from build123d import *

# Parameters (mm, degrees)
F1_DEPTH = 40
F3_DEPTH = 35
F4_R     = 35
F4_R_2   = 2
F5_DEPTH = 5


with BuildPart() as f1:
    # F0 (on Front) → F1 (new body, symmetric)
    with BuildSketch(Plane.XZ):
        Polygon((66.8717782649, 24.1746824527), (40.8910161514, 9.1746824527), (-28.3910161514, -30.8253175473), (-28.3910161514, -40.8253175473), (51.6089838486, -40.8253175473), (51.6089838486, -13.5048094716), (82.2307621135, 4.1746824527), (147.2307621135, 4.1746824527), (147.2307621135, 24.1746824527), align=None)
    extrude(amount=F1_DEPTH, both=True)

    # F2 (on Front) → F3 (cut, symmetric)
    with BuildSketch(Plane.XZ):
        with BuildLine():
            ThreePointArc((-23.4223891848, -30.2660805074), (17.6554756717, -37.2808918374), (50.6089838486, -11.772758664))
            Line((50.6089838486, -11.772758664), (81.6948637287, 6.1746824527))
            Line((81.6948637287, 6.1746824527), (145.2307621135, 6.1746824527))
            Line((145.2307621135, 6.1746824527), (145.2307621135, 12.1746824527))
            ThreePointArc((145.2307621135, 12.1746824527), (142.3018299254, 19.2457502646), (135.2307621135, 22.1746824527))
            Line((135.2307621135, 22.1746824527), (67.4076766498, 22.1746824527))
            Line((67.4076766498, 22.1746824527), (-23.4223891848, -30.2660805074))
        make_face()
    extrude(amount=F3_DEPTH, both=True, mode=Mode.SUBTRACT)

    # F4 (on face) → F5 (cut)
    with BuildSketch(Plane(origin=(6.25, 0, -10.8253175473), x_dir=(0.8660254038, 0, 0.5), z_dir=(-0.5, 0, 0.8660254038))):
        Circle(F4_R)
        with Locations((-35.75, 35.75)):
            Circle(F4_R_2)
        with Locations((35.75, 35.75)):
            Circle(F4_R_2)
        with Locations((35.75, -35.75)):
            Circle(F4_R_2)
        with Locations((-35.75, -35.75)):
            Circle(F4_R_2)
    extrude(amount=-F5_DEPTH, mode=Mode.SUBTRACT)


solid = f1.part
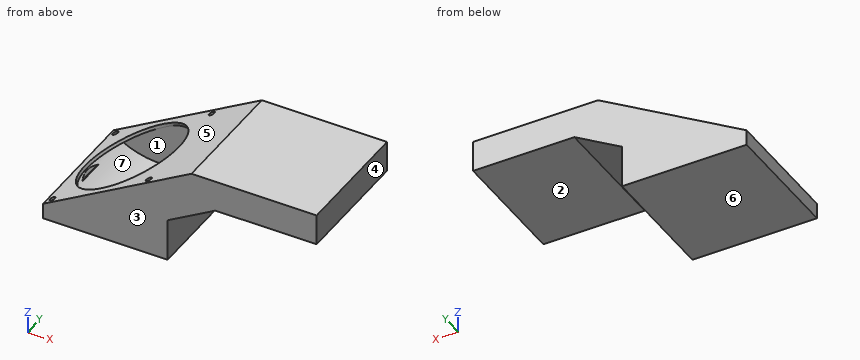
The listing builds one solid part. Answer for the finished solid, in the listing's coordinates (mm). Face numbers are marked on the shaded views. A direction names the side the tool comes from. Coordinates: 2 decimals unless noted, no trailing zeros. Loops run counter-clockwise (first coordinate to the right, second up) from the corner with the lowest first, then second, coordinate; pieces in that order, holes last. Notation, with made-up numbers: (-14, 17.5) -> (-3, 17.5) arc R26 ccw to (-3, 34.5) -> close; hole circle Ø3 at (-9, -11.75). An arc over 180 degrees is marked (long way). Answer in a Markdown table with one row per item. Add a question column.
1. The part is cut by section C-C, the plane y = -13. Write down the section's boundary in (x, z), then the cut area to 3 significant figures.
2. For the marked faces 1, 2 and 3, determine the directions among +Z, -Z, +X, -X, +Y, -Y from which every point of the face is accessible in a straight line to the end or side of a thin tool.
3. The part is cut by section D-D, the plane y = 6.5. Write down the section's boundary in (x, z), then the cut area to 3 significant figures.
4. Consider line 1 (Z direction, x = 105.5, y = -21.5); line 2 (Y direction, x = 45.5, z = -7); line 3 (Y direction, x = 11, z = -10). Determine where each line is inside the solid, lowest interval first. Write a range as [from, to].
5. Flat-ended cylindrical pins translate along their axes: P1, Ø12, axis at x = 37.5, y = -0.5, coming from the +Z side; P2, Ø4, axis at y = -6, z = -19.5, coming from the +X side; P3, Ø3, axis at y = -13, z = 10, coming from the -X side. Find the tip coordinate at first contact, or state that the pin passes through.
6. The part is cut by section A-A, the plane x = 114. Write down the section's boundary in (y, z), then the cut area to 3 significant figures.
7. The part is cut by section B-B, the plane y = 20. Write down the section's boundary in (x, z).
8. Determine the mould class of the marked faces 4, 5, 6 and 7 for opening direction X: +X half, -X half, draft (parallel to the pull), parting line (faces both ways), or undercut.
Answer below:
| question | item | result |
|---|---|---|
| 1 | outline | (-28.39, -40.83) -> (51.61, -40.83) -> (51.61, -13.5) -> (82.23, 4.17) -> (147.23, 4.17) -> (147.23, 24.17) -> (66.87, 24.17) -> (34.39, 5.42) -> (35.39, 3.69) -> (67.41, 22.17) -> (135.23, 22.17) arc R10 cw to (145.23, 12.17) -> (145.23, 6.17) -> (81.69, 6.17) -> (50.61, -11.77) arc R51.8 cw to (-23.42, -30.27) -> (-20.89, -28.81) -> (-21.89, -27.07) -> (-28.39, -30.83) -> close |
| 1 | area | 1,160 mm2 |
| 2 | face 1 | none |
| 2 | face 2 | -Z, +X, +Y, -Y |
| 2 | face 3 | +Z, -Z, +X, -X, -Y |
| 3 | outline | (-28.39, -40.83) -> (51.61, -40.83) -> (51.61, -13.5) -> (82.23, 4.17) -> (147.23, 4.17) -> (147.23, 24.17) -> (66.87, 24.17) -> (36.03, 6.37) -> (37.03, 4.64) -> (67.41, 22.17) -> (135.23, 22.17) arc R10 cw to (145.23, 12.17) -> (145.23, 6.17) -> (81.69, 6.17) -> (50.61, -11.77) arc R51.8 cw to (-20.51, -32.05) -> (-21.03, -32.35) -> (-21.56, -31.44) arc R51.8 cw to (-23.42, -30.27) -> (-22.53, -29.75) -> (-23.53, -28.02) -> (-28.39, -30.83) -> close |
| 3 | area | 1,150 mm2 |
| 4 | line 1 | [4.17, 6.17], [22.17, 24.17] |
| 4 | line 2 | [-40, -35], [35, 40] |
| 4 | line 3 | [-40, -34.71], [34.71, 40] |
| 5 | P1 | z = 10.68 |
| 5 | P2 | x = 51.61 |
| 5 | P3 | x = 39.72 |
| 6 | outline | (-40, 4.17) -> (40, 4.17) -> (40, 24.17) -> (-40, 24.17) -> close; hole (-35, 6.17) -> (35, 6.17) -> (35, 22.17) -> (-35, 22.17) -> close |
| 6 | area | 480 mm2 |
| 7 | outline | (-28.39, -40.83) -> (51.61, -40.83) -> (51.61, -13.5) -> (82.23, 4.17) -> (147.23, 4.17) -> (147.23, 24.17) -> (66.87, 24.17) -> (31.12, 3.54) -> (32.12, 1.8) -> (67.41, 22.17) -> (135.23, 22.17) arc R10 cw to (145.23, 12.17) -> (145.23, 6.17) -> (81.69, 6.17) -> (50.61, -11.77) arc R51.8 cw to (-23.42, -30.27) -> (-17.62, -26.92) -> (-18.62, -25.19) -> (-28.39, -30.83) -> close |
| 8 | face 4 | +X half |
| 8 | face 5 | -X half |
| 8 | face 6 | draft |
| 8 | face 7 | undercut |
